For this review, take the finished solid that the model builds, in its own axes (mm). A direction names the side the tool comes from. Coordinates: 2 decimals unless noted, no trailing zeros. Loops run counter-clockwise (first coordinate to the right, second up) from the corner with the lowest first, then second, coordinate; pieces in that order, holes last. Notation, with made-up numbers: (-28, -26.75) -> (-9, -26.75) arc R34 cw to (-9, 3.25) -> close; hole circle Ø3 at (15, -11.5). An arc over 180 degrees is marked (long way). Answer in a Markdown table with one row per item.
from build123d import *

# Parameters (mm, degrees)
BOSS_EXTRUDE1_DEPTH = 3
SKETCH2_R           = 3.575
CUT_EXTRUDE1_DEPTH  = 3.95
BOSS_EXTRUDE2_DEPTH = 1.64
BOSS_EXTRUDE6_DEPTH = 3
CUT_EXTRUDE8_REACH  = 53.812
SKETCH11_R          = 1


with BuildPart() as part:
    # Sketch1 → Boss-Extrude1 (new body)
    with BuildSketch(Plane(origin=(0, 0, 0), x_dir=(1, 0, 0), z_dir=(0, 1, 0))):
        with BuildLine():
            Line((0, 7), (40, 7))
            Line((40, 7), (40, -7))
            Line((40, -7), (0, -7))
            ThreePointArc((0, -7), (-7, 0), (0, 7))
        make_face()
    extrude(amount=BOSS_EXTRUDE1_DEPTH)

    # Sketch2 → Cut-Extrude1 (cut)
    with BuildSketch(Plane.XZ):
        with Locations(Location((0, 0, 0), (0, 0, 270))):
            Circle(SKETCH2_R)
    extrude(amount=-CUT_EXTRUDE1_DEPTH, mode=Mode.SUBTRACT)

    # Sketch3 → Boss-Extrude2 (add)
    with BuildSketch(Plane(origin=(0, 3, 0), x_dir=(1, 0, 0), z_dir=(0, 1, 0))):
        with BuildLine():
            Line((40, -7), (40, 7))
            Line((40, 7), (0, 7))
            ThreePointArc((0, 7), (-7, 0), (0, -7))
            Line((0, -7), (40, -7))
        make_face()
        with BuildLine():
            Line((14.43004688, 2.119993993), (2.468524523, 2.816276208))
            ThreePointArc((2.468524523, 2.816276208), (-3.745, 0), (2.468524523, -2.816276208))
            Line((2.468524523, -2.816276208), (14.43004688, -2.119993993))
            ThreePointArc((14.43004688, -2.119993993), (16.545, 0), (14.43004688, 2.119993993))
        make_face(mode=Mode.SUBTRACT)
    extrude(amount=BOSS_EXTRUDE2_DEPTH)

    # Sketch9 → Boss-Extrude6 (add)
    with BuildSketch(Plane(origin=(40, 0, 0), x_dir=(0, 0, -1), z_dir=(1, 0, 0))):
        with BuildLine():
            Line((-7, 4.64), (-7, 0))
            Line((-7, 0), (7, 0))
            Line((7, 0), (7, 4.64))
            ThreePointArc((7, 4.64), (0, 11.64), (-7, 4.64))
        make_face()
    extrude(amount=BOSS_EXTRUDE6_DEPTH)

    # Sketch11 → Cut-Extrude8 (cut, up to next)
    with BuildSketch(Plane(origin=(43, 0, 0), x_dir=(0, 0, -1), z_dir=(1, 0, 0)), mode=Mode.PRIVATE) as cut_extrude8_sk1:
        with BuildLine():
            Line((0, 7.554213562), (-0.707106782, 6.84710678))
            ThreePointArc((-0.707106782, 6.84710678), (1e-09, 7.14), (0.707106784, 6.847106778))
            Line((0.707106784, 6.847106778), (0, 7.554213562))
        make_face()
    cut_extrude8_tool1 = extrude(cut_extrude8_sk1.sketch, amount=-CUT_EXTRUDE8_REACH, mode=Mode.PRIVATE) & part.part
    # Sketch11 → Cut-Extrude8 (cut, up to next)
    with BuildSketch(Plane(origin=(43, 0, 0), x_dir=(0, 0, -1), z_dir=(1, 0, 0)), mode=Mode.PRIVATE) as cut_extrude8_sk2:
        with BuildLine():
            ThreePointArc((0.707106779, 5.432893216), (-2e-09, 5.14), (-0.707106782, 5.43289322))
            Line((-0.707106782, 5.43289322), (0, 4.725786438))
            Line((0, 4.725786438), (0.707106779, 5.432893216))
        make_face()
    cut_extrude8_tool2 = extrude(cut_extrude8_sk2.sketch, amount=-CUT_EXTRUDE8_REACH, mode=Mode.PRIVATE) & part.part
    # Sketch11 → Cut-Extrude8 (cut, up to next)
    with BuildSketch(Plane(origin=(43, 0, 0), x_dir=(0, 0, -1), z_dir=(1, 0, 0)), mode=Mode.PRIVATE) as cut_extrude8_sk3:
        with Locations((0, 6.14)):
            Circle(SKETCH11_R)
    cut_extrude8_tool3 = extrude(cut_extrude8_sk3.sketch, amount=-CUT_EXTRUDE8_REACH, mode=Mode.PRIVATE) & part.part
    add(cut_extrude8_tool1.solids().sort_by_distance((43, 7.238324, 0))[0], mode=Mode.SUBTRACT)
    add(cut_extrude8_tool2.solids().sort_by_distance((43, 5.041676, 0))[0], mode=Mode.SUBTRACT)
    add(cut_extrude8_tool3.solids().sort_by_distance((43, 6.14, 0))[0], mode=Mode.SUBTRACT)


solid = part.part
Item 1: For L1, parallel to X at y = 2.2, z = 0 (3 decimals); L2, parallel to Z at x = 0, y = 4 (3 decimals); L3, parallel to Y at x = 10, z = -3.25, list the stretches that pass through material, from the lowest coordinate up.
Worked answers:
| item | result |
|---|---|
| L1 | -7 to -3.575, 3.575 to 43 |
| L2 | -7 to -3.745, 3.745 to 7 |
| L3 | 0 to 4.64 |
Item 2: The part is to be moulded in two halves that separate along Z. For faces 5 (the cylindrical face through (16.544, 3.809, 0.047)), 6 (the flat face through (18, 0, 0)), 7 (the cylindrical face through (41.48, 11.64, -0.15)), 8 (the flat face through (21, 2, 7)), say which applies: +Z half, -Z half, draft (parallel to the pull), parting line (faces both ways), or undercut.
Worked answers:
| item | result |
|---|---|
| face 5 | undercut |
| face 6 | draft |
| face 7 | parting line |
| face 8 | +Z half |
Item 3: Take a section at A-A, the plane x = 34. State the section outline as (y, z) points.
Worked answers:
| item | result |
|---|---|
| outline | (0, -7) -> (4.64, -7) -> (4.64, 7) -> (0, 7) -> close |
Item 4: Take a section at B-B, the plane z = 6.25. State the section outline as (x, y) points, and give its area (3 significant figures).
Worked answers:
| item | result |
|---|---|
| outline | (-3.15, 0) -> (43, 0) -> (43, 7.79) -> (40, 7.79) -> (40, 4.64) -> (-3.15, 4.64) -> close |
| area | 224 mm² |
Item 5: For faces 1 (the cylindrical face through (41.5, 6.1, -1)), 2 (the flat face through (8.366, 3.809, 2.473)), 3 (the flat face through (21, 2, -7)), 4 (the flat face through (21, 4.64, 0)), list the 3-axis set-ups (+Z, -Z, +X, -X, +Y, -Y) from which the entire face can be reached by the end or side of a thin tool; tool diameter is ignored.
Worked answers:
| item | result |
|---|---|
| face 1 | +X, -X |
| face 2 | +Y |
| face 3 | -Z, +X, -X, +Y, -Y |
| face 4 | +Z, -Z, -X, +Y |
Item 6: Insertion check: pin 1 (2 mm diameter, centred on x = 7, z = 1, fed in from +Y); pin 2 (5.5 mm diameter, centred on y = 9.5, z = -0.5, fed in from -X); pin 3 (8 mm diameter, centred on x = 0, z = -0.5, fed in from +Y). Each pin has a flat end and moves straight along its axis. Give the tip position at first contact, or say it passes through.
Worked answers:
| item | result |
|---|---|
| pin 1 | y = 3 |
| pin 2 | x = 40 |
| pin 3 | y = 4.64 |
Item 7: Take a section at C-C, the plane y = 8.5. State the section outline as (x, z) points.
Worked answers:
| item | result |
|---|---|
| outline | (40, -5.84) -> (43, -5.84) -> (43, 5.84) -> (40, 5.84) -> close |
